For this review, use the dimensioned drawing (mm, ordinates from the lowest corner) and the shaded views. A direction names the side the tool comes from. Round coordinates to 2 decimals unless told otherwise and drop trailing zeros. Order: outer loops, then holes, each group sorted by start corner. A loop starts at its lowest first (then second) coordinate and runs counter-clockwise, first axis right, second up. Notation, with made-up numbers: (-6, 75.25) - (0, 75.25) arc R23 cw to (0, 85.25) - close; hole circle Ø4 at (72.5, 29.5). An arc over 180 degrees is marked (long way). Write item = value, one per line.
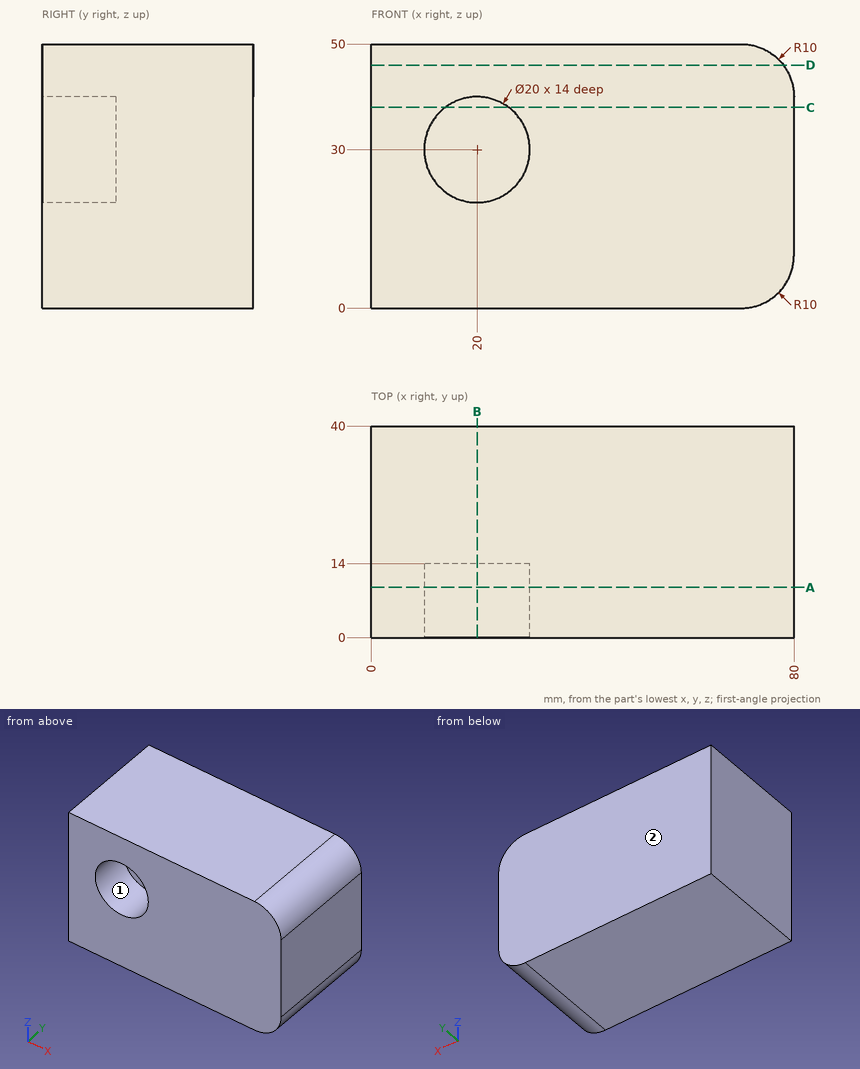
Item 1: For the marked faces 1 and 2, list the 3-axis set-ups (+Z, -Z, +X, -X, +Y, -Y) from which the entire face can be reached by the end or side of a thin tool; tool diameter is ignored.
Data:
face_1 = -Y
face_2 = +Z, -Z, +X, -X, +Y
Item 2: Take a section at D-D, the plane z = 46. State the section outline as (x, y) points.
Data:
outline = (0, 0) - (78, 0) - (78, 40) - (0, 40) - close
Item 3: For line 1 along Z through (x, y) = (20, 6); line 2 along Y through (x, z) = (16.5, 22.5); line 3 along X through (y, z) = (3, 34), list the stretches that pass through material, from the lowest coordinate up. Write a range as [from, to].
Data:
line_1 = [0, 20], [40, 50]
line_2 = [14, 40]
line_3 = [0, 10.83], [29.17, 80]
Item 4: Take a section at B-B, the plane x = 20. State the section outline as (y, z) points.
Data:
outline = (0, 0) - (40, 0) - (40, 50) - (0, 50) - (0, 40) - (14, 40) - (14, 20) - (0, 20) - close
Item 5: Take a section at C-C, the plane z = 38. State the section outline as (x, y) points.
Data:
outline = (0, 0) - (14, 0) - (14, 14) - (26, 14) - (26, 0) - (80, 0) - (80, 40) - (0, 40) - close
Item 6: Take a section at A-A, the plane y = 9.5. State the section outline as (x, z) points.
Data:
outline = (0, 0) - (70, 0) arc R10 ccw to (80, 10) - (80, 40) arc R10 ccw to (70, 50) - (0, 50) - close; hole circle Ø20 at (20, 30)
